Verification items for the finished model (mm, model axes). Face numbers are marked on the shaded views. Coordinates: 2 decimals unless noted, no trailing zeros. Write each loop counter-clockwise with the first axis right and the second up, starting at its lowest first coordinate (ties: lowest second). Pieces come first, ordered by that corner, then holes. Notation, with made-up numbers: (-20.75, -23.75) - (34.25, -23.75) arc R6 cw to (34.25, -14.75) - close; hole circle Ø6 at (46, 55). An arc over 180 degrees is marked (long way). Use one line per item in the form item = value. Start each with the question number.
(1) Material ranges on line 1 (X direction, y = 15, z = -27.5); line 2 (Y direction, x = 0.7, z = 0); line 3 (X direction, y = 17, z = -0.5), recorded low to high. Write a range as [from, to].
(2) Sectioned sample at A-A (z = 0). Count the separate pieces of the cut face and the enclosed holes in it, and give its area (3 significant figures).
(3) Sectioned sample at B-B (x = -128.5). Record the cut outline in (y, z).
(4) Gauge pin test, flat ends, axial feed: pin 1 Ø1.5 at (x, y) = (-40.5, 11.5) entering from +Z; pin 2 Ø2 at (x, z) = (-58, 10) entering from +Y; pin 3 Ø3 at (x, y) = (-76.5, 14.5) entering from +Z; pin 4 Ø18 at (y, z) = (0, 0) entering from +X. Record the tip position at first contact, or that the pin passes through.
(5) Sectioned sample at C-C (y = 5.5). Record the cut outline in (x, z), and give its area (3 significant figures).
(6) Sectioned sample at D-D (x = -164.5). Record the cut outline in (y, z).
(7) Mould release check, pull along X, two halves, no side actions. Record for the marked faces 1 and 2: released by +X, released by -X, zero draft, split by the parting line, or undercut.
Autodesk Inventor part; units mm, degrees
ref_plane "YZ Plane" through (0, 0, 0) normal (1, 0, 0) x (0, 1, 0)
ref_plane "XZ Plane" through (0, 0, 0) normal (0, 1, 0) x (-1, 0, 0)
ref_plane "XY Plane" through (0, 0, 0) normal (0, 0, 1) x (1, 0, 0)
sketch "Sketch1" plane through (0, 0, 0) normal (1, 0, 0) x (0, 1, 0)
  circle A0 centre (0, 0) radius 11.25
  line L0 (-11.25, 11.25) -> (11.25, 11.25) construction
  line L1 (11.25, 11.25) -> (11.25, -11.25) construction
  line L2 (11.25, -11.25) -> (-11.25, -11.25) construction
  line L3 (-11.25, -11.25) -> (-11.25, 11.25) construction
  line L4 (-11.25, 11.25) -> (11.25, -11.25) construction
  line L5 (11.25, 11.25) -> (-11.25, -11.25) construction
  line L6 (11.25, 11.25) -> (14.25, 11.25) construction
  line L7 (14.25, 11.25) -> (14.25, -11.25) construction
  line L8 (14.25, -11.25) -> (11.25, -11.25) construction
  line L9 (11.25, -11.25) -> (11.25, 11.25) construction
  line L10 (14.25, -11.25) -> (-11.25, -11.25) construction
  line L11 (-11.25, -11.25) -> (-11.25, -14.25) construction
  line L12 (-11.25, -14.25) -> (14.25, -14.25) construction
  line L13 (14.25, -14.25) -> (14.25, -11.25) construction
  line L14 (-13, 13) -> (13, 13)
  line L15 (13, 13) -> (13, -13)
  line L16 (13, -13) -> (-13, -13)
  line L17 (-13, -13) -> (-13, 13)
  line L18 (-13, 13) -> (13, -13) construction
  line L19 (13, 13) -> (-13, -13) construction
  dimension "d0" = 22.5
  dimension "d1" = 3
  dimension "d2" = 3
  dimension "d3" = 26
  dimension "d4" = 26
extrude "Extrusion1" add sketch "Sketch1" along normal blind 9
sketch "Sketch2" plane through (0, 0, 0) normal (-1, 0, 0) x (0, 0, 1)
  circle A0 centre (0, 0) radius 7.75
  circle A1 centre (0, 0) radius 11.25
  dimension "d7" = 15.5
extrude "Extrusion2" add sketch "Sketch2" against normal blind 2
sketch "Sketch3" plane through (0, 0, 0) normal (-1, 0, 0) x (0, 0, 1)
  line L0 (13, 13) -> (-13, 13)
  line L1 (13, 13) -> (8.75, 13)
  line L2 (8.75, 13) -> (8.75, -13)
  line L3 (8.75, -13) -> (13, -13)
  line L4 (13, -13) -> (13, 13)
  point P0 (0, 0)
  dimension "d10" = 4.25
  dimension "d11" = 26
extrude "Extrusion3" add sketch "Sketch3" along normal blind 168
sketch "Sketch4" plane through (-168, 0, 0) normal (-1, 0, 0) x (0, 0, 1)
  line L0 (13, 13) -> (13, -13)
  line L1 (-13, -13) -> (-13, 13)
  line L2 (13, -13) -> (-13, -13)
  line L3 (-13, -13) -> (-13, 13)
  line L4 (-13, 13) -> (13, 13)
  line L5 (13, 13) -> (13, -13)
  circle A0 centre (0, 0) radius 7.75
  circle A1 centre (0, 0) radius 11.25
extrude "Extrusion4" add sketch "Sketch4" along normal blind 9 contours L0 L2 L1 L4
sketch "Sketch5" plane through (-168, 0, 0) normal (1, 0, 0) x (0, 0, -1)
  circle A0 centre (0, 0) radius 7.75
  circle A1 centre (0, 0) radius 11.25
extrude "Extrusion5" add sketch "Sketch5" against normal blind 2
sketch "Sketch6" plane through (0, 13, -13) normal (0, 1, 0) x (1, 0, 0)
  line L0 (9, -26) -> (9, 0)
  line L1 (-177, -26) -> (-177, 0)
  line L2 (9, 0) -> (-177, 0)
  line L3 (-177, 0) -> (-177, -26)
  line L4 (-177, -26) -> (9, -26)
  line L5 (9, -26) -> (9, 0)
  point P0 (0, -13)
extrude "Extrusion6" add sketch "Sketch6" along normal blind 5.5
ref_plane "Work Plane1" through (0, 0, 0) normal (-1, 0, 0) x (0, 0, 1)
sketch "Sketch7" plane through (0, 0, 0) normal (-1, 0, 0) x (0, 0, 1)
  line L0 (13, -13) -> (13, 18.5)
  line L1 (13, 18.5) -> (3.75, 18.5)
  line L2 (3.75, 18.5) -> (3.75, 9.5)
  line L3 (3.75, 9.5) -> (13, 9.5)
  line L4 (13, 9.5) -> (13, 18.5)
  point P0 (0, 0)
  dimension "d21" = 9.25
  dimension "d22" = 9
extrude "Extrusion7" cut sketch "Sketch7" along normal blind 168
sketch "Sketch8" plane through (0, 0, 0) normal (-1, 0, 0) x (0, 0, 1)
  point P0 (0, 0)
sketch "Sketch9" plane through (-177, -13, 13) normal (0, 0, 1) x (1, 0, 0)
  point P0 (177, 13)
sketch "Sketch10" plane through (-177, -13, 13) normal (0, 0, 1) x (1, 0, 0)
  line L0 (0, 0) -> (0, 31.5) construction
  line L1 (9, 0) -> (0, 0) construction
  line L2 (0, 31.5) -> (9, 31.5) construction
  line L3 (9, 31.5) -> (9, 0) construction
  line L4 (9, 0) -> (0, 0) construction
  line L5 (0, 0) -> (0, 31.5) construction
  line L6 (186, 31.5) -> (0, 31.5) construction
  line L7 (0, 0) -> (186, 0) construction
  line L8 (186, 31.5) -> (177, 31.5) construction
  line L9 (177, 31.5) -> (177, 0) construction
  line L10 (177, 0) -> (186, 0) construction
  line L11 (186, 0) -> (186, 31.5) construction
  line L12 (9, 22.5) -> (9, 0)
  line L13 (177, 0) -> (177, 22.5)
  line L14 (9, 0) -> (177, 0)
  line L15 (177, 0) -> (177, 9)
  line L16 (177, 9) -> (9, 9)
  line L17 (9, 9) -> (9, 0)
  point P0 (177, 13)
  dimension "d25" = 9
extrude "Extrusion8" cut sketch "Sketch10" against normal blind 5
fillet "Fillet1" radius 6.5 2 edges at (0, -4, 10.875) (-168, -4, 10.875)
sketch "Sketch11" plane through (9, -13, -13) normal (0, 0, -1) x (-1, 0, 0)
  point P0 (9, 13)
sketch "Sketch12" plane through (9, -13, -13) normal (0, 0, -1) x (-1, 0, 0)
  line L0 (0, 31.5) -> (186, 31.5) construction
  line L1 (9, 26) -> (177, 26) construction
  line L2 (0, 31.5) -> (22, 31.5) construction
  line L3 (22, 31.5) -> (22, 26) construction
  line L4 (22, 26) -> (0, 26) construction
  line L5 (0, 26) -> (0, 31.5) construction
  line L6 (17.1, 27.15) -> (4.9, 27.15) construction
  line L7 (4.9, 27.15) -> (4.9, 30.35) construction
  line L8 (4.9, 30.35) -> (17.1, 30.35) construction
  line L9 (17.1, 30.35) -> (17.1, 27.15) construction
  line L10 (17.1, 27.15) -> (4.9, 30.35) construction
  line L11 (4.9, 27.15) -> (17.1, 30.35) construction
  line L12 (17.1, 27.15) -> (4.9, 27.15)
  line L13 (4.9, 27.15) -> (4.9, 30.35)
  line L14 (4.9, 30.35) -> (17.1, 30.35)
  line L15 (17.1, 30.35) -> (17.1, 27.15)
  line L16 (17.1, 27.15) -> (4.9, 30.35) construction
  line L17 (4.9, 27.15) -> (17.1, 30.35) construction
  line L18 (186, 0) -> (186, 31.5) construction
  line L19 (186, 31.5) -> (164, 31.5) construction
  line L20 (164, 31.5) -> (164, 26) construction
  line L21 (164, 26) -> (186, 26) construction
  line L22 (186, 26) -> (186, 31.5) construction
  line L23 (181.1, 27.15) -> (168.9, 27.15)
  line L24 (168.9, 27.15) -> (168.9, 30.35)
  line L25 (168.9, 30.35) -> (181.1, 30.35)
  line L26 (181.1, 30.35) -> (181.1, 27.15)
  line L27 (181.1, 27.15) -> (168.9, 30.35) construction
  line L28 (168.9, 27.15) -> (181.1, 30.35) construction
  line L29 (22, 26) -> (0, 26)
  line L30 (0, 26) -> (0, 31.5)
  line L31 (0, 31.5) -> (22, 31.5)
  line L32 (22, 31.5) -> (22, 26)
  line L33 (164, 26) -> (186, 26)
  line L34 (186, 26) -> (186, 31.5)
  line L35 (186, 31.5) -> (164, 31.5)
  line L36 (164, 31.5) -> (164, 26)
  point P0 (9, 13)
  point P1 (11, 28.75)
  point P2 (175, 28.75)
  dimension "d29" = 22
  dimension "d30" = 12.2
  dimension "d31" = 3.2
  dimension "d32" = 22
  dimension "d33" = 12.2
  dimension "d34" = 3.2
extrude "Extrusion9" add sketch "Sketch12" along normal blind 40
sketch "Sketch13" plane through (4.1, 17.35, -13) normal (0, 0, -1) x (-1, 0, 0)
  line L0 (0, 0) -> (12.2, 0)
  line L1 (0, -3.2) -> (12.2, -3.2)
  line L2 (0, 0) -> (12.2, 0)
  line L3 (12.2, 0) -> (12.2, -3.2)
  line L4 (12.2, -3.2) -> (0, -3.2)
  line L5 (0, -3.2) -> (0, 0)
  line L6 (176.2, 0) -> (164, 0)
  line L7 (164, -3.2) -> (176.2, -3.2)
  line L8 (164, 0) -> (176.2, 0)
  line L9 (176.2, 0) -> (176.2, -3.2)
  line L10 (176.2, -3.2) -> (164, -3.2)
  line L11 (164, -3.2) -> (164, 0)
  point P0 (4.1, -17.35)
extrude "Extrusion10" cut sketch "Sketch13" against normal blind 15
sketch "Sketch14" plane through (-177, 0, 0) normal (-1, 0, 0) x (0, 0, 1)
  line L0 (14, -14) -> (-14, -14) construction
  line L1 (-14, -14) -> (-14, 14) construction
  line L2 (-14, 14) -> (14, 14) construction
  line L3 (14, 14) -> (14, -14) construction
  line L4 (14, -14) -> (-14, 14) construction
  line L5 (-14, -14) -> (14, 14) construction
  point P0 (0, 0)
  dimension "d39" = 28
  dimension "d40" = 28
sketch "Sketch15" plane through (0, 0, 0) normal (-1, 0, 0) x (0, 0, 1)
  line L0 (-33, -19) -> (-14, -19) construction
  line L1 (-14, -19) -> (-14, 0) construction
  line L2 (-33, 19) -> (-14, 19) construction
  line L3 (-14, -19) -> (-52, -19) construction
  line L4 (-52, -19) -> (-52, 19) construction
  line L5 (-52, 19) -> (-14, 19) construction
  point P0 (0, 0)
  dimension "d41" = 19
  dimension "d45" = 38
properties part number "rearAxelHolder 9-19"
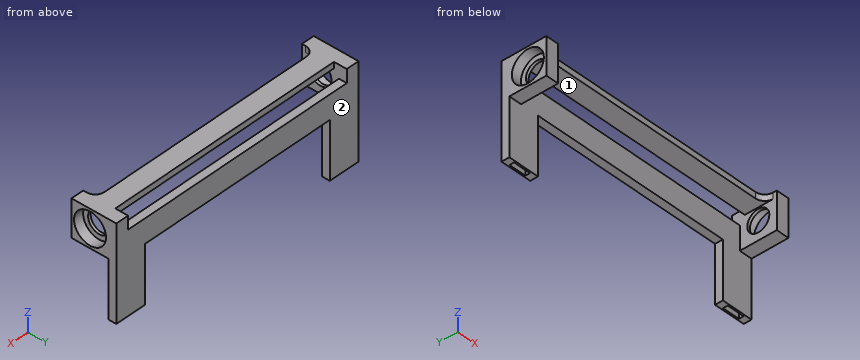
Answers below:
q1.line_1 = [-177, -172.1], [-159.9, -155], [-13, -8.1], [4.1, 9]
q1.line_2 = [-13, -7.75], [7.75, 14.15], [17.35, 18.5]
q1.line_3 = [-177, -172.1], [-159.9, -8.1], [4.1, 9]
q2.separate_pieces = 3
q2.enclosed_holes = 2
q2.area = 1,040 mm2
q3.outline = (-4, 8.75) - (9.5, 8.75) - (9.5, 13) - (-4, 13) - close; (13, -13) - (18.5, -13) - (18.5, 3.75) - (13, 3.75) - close
q4.pin_1 = through
q4.pin_2 = 9.5
q4.pin_3 = 3.75
q4.pin_4 = 2
q5.outline = (-177, -13) - (-168, -13) - (-168, -5.46) - (-170, -5.46) - (-170, -9.81) - (-177, -9.81) - close; (-177, 9.81) - (-170, 9.81) - (-170, 5.46) - (-168, 5.46) - (-168, 8.75) - (0, 8.75) - (0, 5.46) - (2, 5.46) - (2, 9.81) - (9, 9.81) - (9, 13) - (-177, 13) - close; (0, -13) - (9, -13) - (9, -9.81) - (2, -9.81) - (2, -5.46) - (0, -5.46) - close
q5.area = 864 mm2
q6.outline = (-4.73, 8.75) - (9.5, 8.75) - (9.5, 13) - (-4.73, 13) - close; (13, -53) - (14.15, -53) - (14.15, 2) - (17.35, 2) - (17.35, -53) - (18.5, -53) - (18.5, 3.75) - (13, 3.75) - close
q7.face_1 = undercut
q7.face_2 = zero draft
